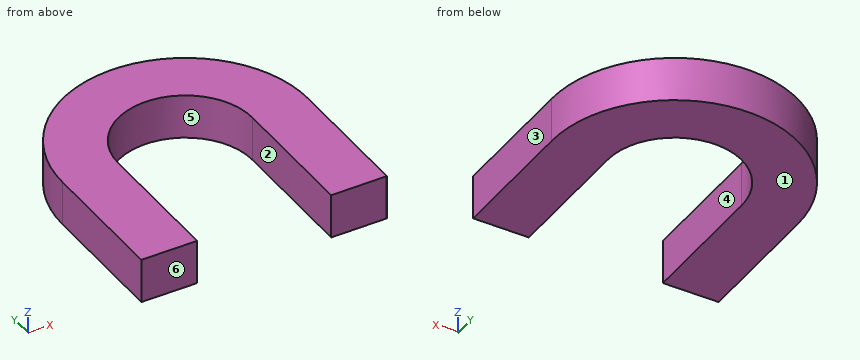
```python
from build123d import *

# Parameters (mm, degrees)
BOSS_EXTRUDE1_DEPTH = 4


with BuildPart() as part:
    # Sketch2 → Boss-Extrude1 (new body)
    with BuildSketch(Plane.XY):
        with BuildLine():
            Line((-37.411863854, 35.187534323), (-37.411863854, 23.187534323))
            Line((-37.411863854, 23.187534323), (-37.440640728, 23.209290717))
            Line((-37.440640728, 23.209290717), (-42.411863854, 23.187534323))
            Line((-42.411863854, 23.187534323), (-42.411863854, 35.187534323))
            ThreePointArc((-42.411863854, 35.187534323), (-48.411863854, 41.187534323), (-54.411863854, 35.187534323))
            Line((-54.411863854, 35.187534323), (-54.411863854, 23.187534323))
            Line((-54.411863854, 23.187534323), (-59.411863854, 23.187534323))
            Line((-59.411863854, 23.187534323), (-59.411863854, 35.187534323))
            ThreePointArc((-59.411863854, 35.187534323), (-48.411863854, 46.187534323), (-37.411863854, 35.187534323))
        make_face()
    extrude(amount=BOSS_EXTRUDE1_DEPTH)


solid = part.part
```
The listing builds one solid part. Answer for the finished solid, in the listing's coordinates (mm). Face numbers are marked on the shaded views. A direction names the side the tool comes from. Give positions to 0.01 mm unless a question says otherwise; leave off trailing zeros. Order: outer loops, then holes, each group sorted by start corner. A loop starts at its lowest first (then second) coordinate and runs counter-clockwise, first axis right, second up. Notation, with made-up numbers: (89, 72.5) -> (133, 72.5) arc R8 ccw to (133, 76.5) -> close; hole circle Ø8 at (-37.5, 72). An arc over 180 degrees is marked (long way). Answer as a JSON object with one key per item and string values. Group by question number.
Item 1: A flat-ended cylindrical pin translates along its axis: pin 1 (8 mm diameter, centred on x = -48, y = 25.5, fed in from +Z). Find the tip coordinate at first contact, or state that the pin passes through.
Item 2: Consider L1, parallel to X at y = 26.5, z = 1.6; L2, parallel to X at y = 38.25, z = 1.8; L3, parallel to Y at x = -48.5, z = 1.05. Determine where each line is inside the solid, lowest interval first. Write a range as from..to.
Item 3: The part is cut by section D-D on x = -44. Write down the section's boundary in (y, z), and give its area (3 significant figures).
Item 4: The part is cut by section C-C on y = 35.75. Write down the section's boundary in (x, z).
Item 5: The part is cut by section A-A on y = 32. Write down the section's boundary in (x, z), and give its area (3 significant figures).
Item 6: Determine the mould class of the marked faces 3, 4, 5 and 6 for opening direction X: pulls with the +X half, pulls with the -X half, needs draft (parallel to the pull), parting line crosses it, or undercut.
Item 7: A tool of negligible diameter and unlimited length cuts with its end or side. For the marked faces 1 and 2, from which of +Z, -Z, +X, -X, +Y, -Y can it reach the whole face along a straight path? Write none if from no direction.
Result set:
{
 "1": {"pin 1": "through"},
 "2": {"L1": "-59.41..-54.41, -42.41..-37.41", "L2": "-58.98..-53.57, -43.25..-37.85", "L3": "41.19..46.19"},
 "3": {"outline": "(39.25, 0) -> (45.26, 0) -> (45.26, 4) -> (39.25, 4) -> close", "area": "24.0 mm²"},
 "4": {"outline": "(-59.4, 0) -> (-54.39, 0) -> (-54.39, 4) -> (-59.4, 4) -> close; (-42.44, 0) -> (-37.43, 0) -> (-37.43, 4) -> (-42.44, 4) -> close"},
 "5": {"outline": "(-59.41, 0) -> (-54.41, 0) -> (-54.41, 4) -> (-59.41, 4) -> close; (-42.41, 0) -> (-37.41, 0) -> (-37.41, 4) -> (-42.41, 4) -> close", "area": "40.0 mm²"},
 "6": {"face 3": "pulls with the +X half", "face 4": "undercut", "face 5": "undercut", "face 6": "needs draft"},
 "7": {"face 1": "-Z, +X, -X, +Y, -Y", "face 2": "+Z, -Z, -Y"}
}
